```python
from build123d import *

# Parameters (mm, degrees)
SKETCH_1_R               = 21
EXTRUDE_1_DEPTH          = 13.7
SKETCH_3_R               = 21
SKETCH_2_R               = 18.3
CUT_EXTRUDE_START        = -4
CUT_EXTRUDE_1_DEPTH      = 4
PATTERN_CIRCULAR_1_COUNT = 12
SKETCH_5_R               = 18.3
EXTRUDE_2_DEPTH          = 1.1
EXTRUDE_3_DEPTH          = 5
SKETCH_8_R               = 3
EXTRUDE_4_DEPTH          = 4
SKETCH_9_R               = 1.1
CUT_EXTRUDE_3_DEPTH      = 4


with BuildPart() as part:
    # 草图1 → 凸台-拉伸1 (new body)
    with BuildSketch(Plane.XY):
        with Locations(Location((0, 0, 0), (0, 0, 191.095408705))):
            Circle(SKETCH_1_R)
    extrude(amount=EXTRUDE_1_DEPTH)

    # 草图3 → 放样1 section 0
    with BuildSketch(Plane.XY.offset(13.7)):
        Circle(SKETCH_3_R)
    # 草图2 → 放样1 section 1
    with BuildSketch(Plane.XY.offset(17.7)):
        Circle(SKETCH_2_R)
    loft()

    # 草图4 → 切除-拉伸1 (cut)
    with BuildSketch(Plane.XY.offset(17.7).offset(CUT_EXTRUDE_START)):
        with BuildLine():
            ThreePointArc((6.924234277, 1.027122038), (6.981032873, 0.51495634), (7, 0))
            Line((7, 0), (18.3, 0))
            ThreePointArc((18.3, 0), (18.217281615, 1.738001882), (17.969874258, 3.460291774))
            Line((17.969874258, 3.460291774), (6.924234277, 1.027122038))
        make_face()
        with BuildLine():
            Line((18.3, 0), (7, 0))
            ThreePointArc((7, 0), (6.981032873, -0.51495634), (6.924234277, -1.027122038))
            Line((6.924234277, -1.027122038), (17.969874258, -3.460291774))
            ThreePointArc((17.969874258, -3.460291774), (18.217281615, -1.738001882), (18.3, 0))
        make_face()
        with BuildLine():
            ThreePointArc((17.969874258, 3.460291774), (18.217281615, 1.738001882), (18.3, 0))
            Line((18.3, 0), (21, 0))
            ThreePointArc((21, 0), (20.9016371, 2.030164166), (20.607469853, 4.041309967))
            Line((20.607469853, 4.041309967), (17.969874258, 3.460291774))
        make_face()
        with BuildLine():
            Line((21, 0), (18.3, 0))
            ThreePointArc((18.3, 0), (18.217281615, -1.738001882), (17.969874258, -3.460291774))
            Line((17.969874258, -3.460291774), (20.607469853, -4.041309967))
            ThreePointArc((20.607469853, -4.041309967), (20.9016371, -2.030164166), (21, 0))
        make_face()
    cut_extrude_1 = extrude(amount=CUT_EXTRUDE_1_DEPTH, mode=Mode.SUBTRACT)

    # 阵列(圆周)1: 切除-拉伸1 ×12 about axis
    pattern_circular_1_axis = Axis((0, 0, 0), (0, 0, -1))
    for i in range(1, PATTERN_CIRCULAR_1_COUNT):
        add(cut_extrude_1.rotate(pattern_circular_1_axis, i * 360 / PATTERN_CIRCULAR_1_COUNT), mode=Mode.SUBTRACT)

    # 草图5 → 凸台-拉伸2 (add)
    with BuildSketch(Plane.XY.offset(17.7)):
        Circle(SKETCH_5_R)
    extrude(amount=-EXTRUDE_2_DEPTH)

    # 草图6 → 凸台-拉伸3 (add)
    with BuildSketch(Plane.XY.offset(17.7)):
        with BuildLine():
            Line((-2.753137561, 2.161072319), (1.303750909, 3.248112308))
            ThreePointArc((1.303750909, 3.248112308), (0.905866658, -3.380740392), (-2.753137561, 2.161072319))
        make_face()
    extrude(amount=EXTRUDE_3_DEPTH)

    # 草图8 → 凸台-拉伸4 (add)
    with BuildSketch(Plane.XY.offset(17.7)):
        with Locations((6.278517871, 1.682323793)):
            Circle(SKETCH_8_R)
        with Locations((-6.278517871, -1.682323793)):
            Circle(SKETCH_8_R)
    extrude(amount=-EXTRUDE_4_DEPTH)

    # 草图9 → 切除-拉伸3 (cut)
    with BuildSketch(Plane.XY.offset(17.7)):
        with Locations((6.278517871, 1.682323793)):
            Circle(SKETCH_9_R)
        with Locations((-6.278517871, -1.682323793)):
            Circle(SKETCH_9_R)
    extrude(amount=-CUT_EXTRUDE_3_DEPTH, mode=Mode.SUBTRACT)


solid = part.part
```
For this review, take the finished solid that the model builds, in its own axes (mm). A direction names the side the tool comes from. Coordinates: 2 decimals unless noted, no trailing zeros. Write each loop counter-clockwise with the first axis right and the second up, starting at its lowest first coordinate (ties: lowest second). Pieces come first, ordered by that corner, then holes. Notation, with made-up numbers: (-13, -31) - (12, -31) arc R24 cw to (12, -9) - close; hole circle Ø11 at (6, -28.75). An arc over 180 degrees is marked (long way). Answer in a Markdown table with one row per item. Add a question column.
Q1. Tool access review of faces 5 (the cylindrical face through (18.3, 0, 17.2)), 6 (the flat face through (0, -14, 16.6)), 7 (the flat face through (8, 13, 13.7)): name each direction out of +Z, -Z, +X, -X, +Y, -Y from which nothing blocks a thin tool from reaching the whole face with its end or side.
Q2. Draft analysis for pull direction X (two halves, no side actions). For faces 1 (the conical face through (-5.062, 18.967, 15.728)), 2 (the flat face through (0, 15, 13.7)), 3 (the flat face through (6, 2, 13.7)), 4 (the conical face through (13.867, -13.895, 15.728)), state which applies: +X half, -X half, draft (parallel to the pull), parting line (faces both ways), or undercut.
Q3. For probe 1 along Z at (x, y) = (-5, 12); probe 2 along X at (y, z) = (-13.5, 16); probe 3 along Z at (x, y) = (9, 8.5), list the stretches that pass through material, from the lowest coordinate up.
Q4. For P1, Ø4, axis at x = 14.5, z = 5, coming from the -Y side; P2, Ø4, axis at x = 7.5, y = 6, coming from the +Z side; P3, Ø6, axis at y = 2.5, z = 16, coming from the -X side, all flat-tipped, find the tip position at first contact; note any pin that passes through.
Q5. We need section A-A, the plane y = 0. State the section outline as (x, z) points.
Q6. We need section D-D, the plane z = 20.75. State the section outline as (x, y) points.
Q7. We need section C-C, the plane y = -12.5. Count the separate pieces of the cut face and the enclosed holes in it, and give its area (3 significant figures).
Q8. We need section B-B, the plane z = 13. State the section outline as (x, y) points.
Answer list:
| question | item | result |
|---|---|---|
| 1 | face 5 | +Z, +X |
| 1 | face 6 | -Y |
| 1 | face 7 | none |
| 2 | face 1 | -X half |
| 2 | face 2 | undercut |
| 2 | face 3 | undercut |
| 2 | face 4 | +X half |
| 3 | probe 1 | z = 0 to 13.7, 16.6 to 17.7 |
| 3 | probe 2 | x = -14 to -11.68, -4.79 to -2.48, 2.48 to 4.79, 11.68 to 14 |
| 3 | probe 3 | z = 0 to 17.7 |
| 4 | P1 | stops at y = -16.87 |
| 4 | P2 | stops at z = 17.7 |
| 4 | P3 | stops at x = -20.99 |
| 5 | outline | (-21, 0) - (21, 0) - (21, 13.7) - (8.76, 13.7) - (8.76, 16.6) - (18.3, 16.6) - (18.3, 17.7) - (3.5, 17.7) - (3.5, 22.7) - (-3.5, 22.7) - (-3.5, 17.7) - (-18.3, 17.7) - (-18.3, 16.6) - (-8.76, 16.6) - (-8.76, 13.7) - (-21, 13.7) - close |
| 6 | outline | (-2.75, 2.16) arc R3.5 ccw (long way) to (1.3, 3.25) - close |
| 7 | separate pieces | 1 |
| 7 | enclosed holes | 3 |
| 7 | area | 527 mm2 |
| 8 | outline | circle Ø42 at (0, 0) |
